Check sheet for the modelled part. Datum: model origin and axes. Units: mm. Face numbers are marked on the shaded views. Round coordinates to 2 decimals unless told otherwise and drop trailing zeros. Order: outer loops, then holes, each group sorted by start corner. A loop starts at its lowest first (then second) coordinate and runs counter-clockwise, first axis right, second up.
Q1. Cross-section at D-D on z = 135. Record the cut outline in (x, y), then the cut area to 3 significant figures.
Q2. Mould release check, pull along Y, two halves, no side actions. Record for the marked faces 1, 2 and 3: +Y half, -Y half, draft (parallel to the pull), parting line (faces both ways), or undercut.
Q3. Scan lines: probe 1 along Z at (x, y) = (90.25, -228); probe 2 along Z at (x, y) = (90.35, -211.5); probe 3 along Y at (x, z) = (95, 287). Record each from-to range of solid material in increasing order.
Q4. Depth check by flat-ended pin: P1, Ø8, axis at x = 122, z = 346.5, coming from the -Y side; P2, Ø2, axis at y = -278, z = 290.5, coming from the +X side; P3, Ø0.6, axis at y = -332, z = 238, coming from the +X side; P4, Ø4.5, axis at y = -178, z = 380, coming from the +X side. Enter the tip coordinate at first touch or a pass-through.
Q5. Cross-section at A-A on z = 48. Record the cut outline in (x, y), then the cut area to 3 significant figures.
Q6. Cross-section at C-C on x = 123.5. Record the cut outline in (y, z).
Q7. Cross-section at B-B on y = -292. Record the cut outline in (x, z), then the cut area to 3 significant figures.
from build123d import *

# Parameters (mm, degrees)
SM_BASE_FLANGE_1_DEPTH           = 400
HOLE_WIZARD_5_2_5_2_1_AT_2_COUNT = 2
HOLE_WIZARD_5_2_5_2_1_AT_2_PITCH = 50
CUT_EXTRUDE_1_DEPTH              = 523.587791668
HOLE_WIZARD_6_0_6_1_D            = 6
HOLE_WIZARD_6_0_6_1_DEPTH        = 220
HOLE_WIZARD_6_0_6_1_TIP          = 1.802581857
SKETCH_11_W                      = 32.021510722
SKETCH_11_H                      = 35
CUT_EXTRUDE_2_DEPTH              = 25


# Sheet-metal steps are written as plain solids
with BuildPart() as part:
    # Sketch 1 → 基体-法兰1 (new body)
    with BuildSketch(Plane.XY):
        with BuildLine():
            Line((136, -146), (91.7366, -146))
            ThreePointArc((91.7366, -146), (91.215745145, -146.215745145), (91, -146.7366))
            Line((91, -146.7366), (91, -330.2634))
            ThreePointArc((91, -330.2634), (91.215745145, -330.784254855), (91.7366, -331))
            Line((91.7366, -331), (100.527645566, -331))
            Line((100.527645566, -331), (100.527645566, -333))
            Line((100.527645566, -333), (91.7366, -333))
            ThreePointArc((91.7366, -333), (89.801531583, -332.198468417), (89, -330.2634))
            Line((89, -330.2634), (89, -146.7366))
            ThreePointArc((89, -146.7366), (89.801531583, -144.801531583), (91.7366, -144))
            Line((91.7366, -144), (136, -144))
            Line((136, -144), (136, -146))
        make_face()
    extrude(amount=SM_BASE_FLANGE_1_DEPTH)

    # 草图6 → Ø5.2 (5.2) 直径孔1 (revolve, cut)
    with BuildSketch(Plane(origin=(89, -178, 380), x_dir=(0, 0, 1), z_dir=(0, 1, 0))):
        Polygon((0, 0), (0, 11.562237609), (2.6, 10), (2.6, 0), align=None)
    hole_wizard_5_2_5_2_1 = revolve(axis=Axis((82.65, -178, 380), (1, 0, 0)), mode=Mode.SUBTRACT)

    # Ø5.2 (5.2) 直径孔1 at 2: Ø5.2 (5.2) 直径孔1 ×2
    with Locations(*[(0, -i * HOLE_WIZARD_5_2_5_2_1_AT_2_PITCH, 0) for i in range(1, HOLE_WIZARD_5_2_5_2_1_AT_2_COUNT)]):
        add(hole_wizard_5_2_5_2_1, mode=Mode.SUBTRACT)

    # 镜向1: Ø5.2 (5.2) 直径孔1 across plane
    add(hole_wizard_5_2_5_2_1.mirror(Plane(origin=(0, 0, 200), x_dir=(1, 0, 0), z_dir=(0, 0, -1))), mode=Mode.SUBTRACT)

    # 镜向1 copy 1 sketch → 镜向1 copy 1 (revolve, cut)
    with BuildSketch(Plane(origin=(89, -228, 20), x_dir=(0, 0, -1), z_dir=(0, 1, 0))):
        Polygon((0, 0), (0, -11.562237609), (2.6, -10), (2.6, 0), align=None)
    revolve(axis=Axis((82.65, -228, 20), (-1, 0, 0)), mode=Mode.SUBTRACT)

    # 草图8 → 切除-拉伸1 (cut, symmetric)
    with BuildSketch(Plane.ZY.offset(-89)):
        Polygon((-267.508163369, -941.508163369), (334.373798762, -339.626201238), (400, -274), (1001.88196213, 327.88196213), (2205.645886391, -875.88196213), (936.255760892, -2145.27208763), align=None)
    cut_extrude_1 = extrude(amount=CUT_EXTRUDE_1_DEPTH, both=True, mode=Mode.SUBTRACT)

    # 镜向2: 切除-拉伸1 across plane
    add(cut_extrude_1.mirror(Plane(origin=(0, 0, 200), x_dir=(1, 0, 0), z_dir=(0, 0, -1))), mode=Mode.SUBTRACT)

    # Ø6.0 (6) 直径孔1
    with Locations(Plane.ZY.offset(-89)):
        with Locations((17, -211.5), (383, -211.5)):
            Hole(HOLE_WIZARD_6_0_6_1_D / 2, depth=HOLE_WIZARD_6_0_6_1_DEPTH)
            with Locations((0, 0, -(HOLE_WIZARD_6_0_6_1_DEPTH + HOLE_WIZARD_6_0_6_1_TIP / 2))):  # 118° drill point
                Cone(0, HOLE_WIZARD_6_0_6_1_D / 2, HOLE_WIZARD_6_0_6_1_TIP, mode=Mode.SUBTRACT)

    # 草图11 → 切除-拉伸2 (cut)
    with BuildSketch(Plane(origin=(0, -144, 0), x_dir=(1, 0, 0), z_dir=(0, 1, 0))):
        with Locations((127.010755361, -390.5)):
            Rectangle(SKETCH_11_W, SKETCH_11_H)
    extrude(amount=-CUT_EXTRUDE_2_DEPTH, mode=Mode.SUBTRACT)


solid = part.part
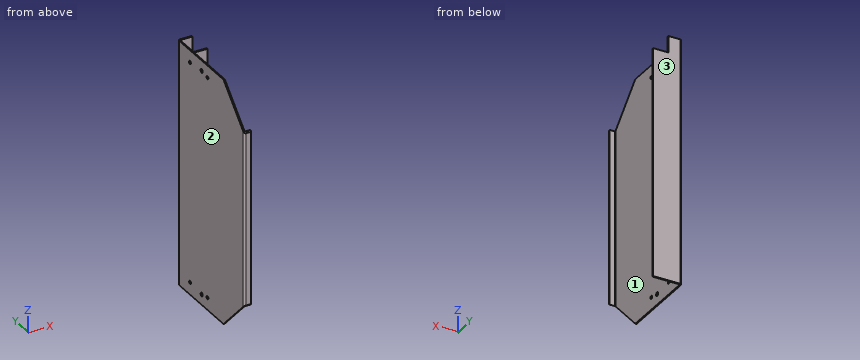
Results found:
1. outline: (89, -330.26) arc R2.74 ccw to (91.74, -333) - (100.53, -333) - (100.53, -331) - (91.74, -331) arc R0.74 cw to (91, -330.26) - (91, -146.74) arc R0.74 cw to (91.74, -146) - (136, -146) - (136, -144) - (91.74, -144) arc R2.74 ccw to (89, -146.74) - close
1. area: 484 mm2
2. face 1: undercut
2. face 2: draft
2. face 3: +Y half
3. probe 1: z = 0 to 17.4, 22.6 to 377.4, 382.6 to 400
3. probe 2: z = 0 to 14, 20 to 380, 386 to 400
3. probe 3: y = -333 to -331, -146 to -144
4. P1: stops at y = -146
4. P2: stops at x = 91
4. P3: stops at x = 100.53
4. P4: passes through
5. outline: (89, -322) - (91, -322) - (91, -146.74) arc R0.74 cw to (91.74, -146) - (136, -146) - (136, -144) - (91.74, -144) arc R2.74 ccw to (89, -146.74) - close
5. area: 445 mm2
6. outline: (-146, 0) - (-144, 0) - (-144, 373) - (-146, 373) - close
7. outline: (89, 18) - (91, 18) - (91, 382) - (89, 382) - close
7. area: 728 mm2
